Autodesk Inventor part; units mm, degrees
ref_plane "YZ Plane" through (0, 0, 0) normal (1, 0, 0) x (0, 1, 0)
ref_plane "XZ Plane" through (0, 0, 0) normal (0, 1, 0) x (-1, 0, 0)
ref_plane "XY Plane" through (0, 0, 0) normal (0, 0, 1) x (1, 0, 0)
sketch "Sketch2" plane through (0, 0, 0) normal (0, 0, 1) x (1, 0, 0)
  line L0 (-43.942, 43.18) -> (-43.942, 15.24)
  line L1 (-43.942, 15.24) -> (-36.322, 15.24)
  line L2 (-36.322, 15.24) -> (-25.4, 0)
  line L3 (-25.4, 0) -> (0, 0)
  line L4 (0, 0) -> (0, 43.18)
  line L5 (0.889, 43.18) -> (0.889, -1.778)
  line L6 (0.889, -1.778) -> (-45.72, -1.778)
  line L7 (-45.72, -1.778) -> (-45.72, 43.18)
  line L8 (-45.72, 43.18) -> (-43.942, 43.18)
  line L9 (0, 43.18) -> (0.889, 43.18)
  dimension "d1" = 7.62
  dimension "d2" = 27.94
  dimension "d3" = 10.922
  dimension "d4" = 43.18
  dimension "d5" = 1.778
  dimension "d6" = 0.889
  dimension "d7" = 1.778
  dimension "d10" = 44.958
  dimension "d11" = 46.609
extrude "Extrusion1" add sketch "Sketch2" along normal mid plane 20.828
sketch "Sketch5" plane through (0.889, -1.778, 10.414) normal (1, 0, 0) x (0, 0, -1)
  line L0 (0, 44.958) -> (20.828, 44.958)
  line L1 (3.175, 44.958) -> (17.653, 44.958)
  line L2 (17.653, 44.958) -> (17.653, 1.778)
  line L3 (17.653, 1.778) -> (3.175, 1.778)
  line L4 (3.175, 1.778) -> (3.175, 44.958)
  line L5 (0, 1.778) -> (20.828, 1.778)
  line L6 (0, 44.958) -> (20.828, 1.778) construction
  line L7 (3.175, 1.778) -> (17.653, 44.958) construction
  point P0 (10.414, 1.778)
  point P1 (10.414, 23.368)
  dimension "d14" = 14.478
extrude "Extrusion2" cut sketch "Sketch5" against normal up to next
sketch "Sketch6" plane through (0, 0, 10.414) normal (0, 0, 1) x (1, 0, 0)
  line L0 (-45.72, 43.18) -> (0.889, 43.18)
  line L1 (0.889, 43.18) -> (0.889, -1.778)
  line L2 (0.889, -1.778) -> (-45.72, -1.778)
  line L3 (-45.72, -1.778) -> (-45.72, 43.18)
extrude "Extrusion3" add sketch "Sketch6" along normal blind 0.889
mirror "Mirror1" about plane through (0, 0, 0) normal (0, 0, 1) of "Extrusion3"
properties part number "SteerServoInsert"
Geometry: final body of the model. Coordinates: model frame, mm. A direction names the side the tool comes from. Round coordinates to 2 decimals unless told otherwise and drop trailing zeros. Write each loop counter-clockwise with the first axis right and the second up, starting at its lowest first coordinate (ties: lowest second). Pieces come first, ordered by that corner, then holes. Notation, with made-up numbers: (11, 6) -> (27, 6) arc R25 cw to (27, 39) -> close; hole circle Ø9 at (-33.5, 12). An arc over 180 degrees is marked (long way). Use CSV: the item, a comma, the result in double quotes. Start each with the question number.
Q1. Section A-A (z = 9). Return loops of the section in (x, y).
Q2. Reachability of faces 4 (the face through (-22, 22, -10.414)), 5 (the face through (-22, 21, -11.303)) from +Z, -Z, +X, -X, +Y, -Y: full face, straight path, thin tool, end or side. Return the list, or none.
Q3. First-contact query: pin 1 Ø6 at (y, z) = (29, 4) entering from +X; pin 2 Ø4 at (x, z) = (-40.5, -0.5) entering from +Y. Flat tips, straight axial feed; report the tip coordinate or a pass-through.
Q4. Section C-C (x = -19). Return loops of the section in (y, z), plus the area to 3 significant figures.
Q5. Line query: L1, parallel to Z at x = -21, y = 38; L2, parallel to X at y = 24.5, z = 9.5; L3, parallel to X at y = 23.5, z = -7. Output: solid intervals per line, ascending.
Q6. Section D-D (z = 2.25). Return loops of the section in (x, y), plus the area to 3 significant figures.
Q7. Section B-B (y = 40). Return loops of the section in (x, z).
Q8. Pull-direction query (X, two-part tool) for faces 1 (the face through (-43.942, 29, 0)), 2 (the face through (0.889, 20, 8)), 3 (the face through (-23, -1.778, 0)); classes: pulls with the +X half, pulls with the -X half, needs draft (parallel to the pull), parting line crosses it, or undercut.
Result sheet:
1,outline,"(-45.72, -1.78) -> (0.89, -1.78) -> (0.89, 43.18) -> (0, 43.18) -> (0, 0) -> (-25.4, 0) -> (-36.32, 15.24) -> (-43.94, 15.24) -> (-43.94, 43.18) -> (-45.72, 43.18) -> close"
2,face 4,"+Y"
2,face 5,"-Z, +X, -X, +Y, -Y"
3,pin 1,"x = -43.94"
3,pin 2,"y = 15.24"
4,outline,"(-1.78, -11.3) -> (43.18, -11.3) -> (43.18, -10.41) -> (0, -10.41) -> (0, 10.41) -> (43.18, 10.41) -> (43.18, 11.3) -> (-1.78, 11.3) -> close"
4,area,"117 mm²"
5,L1,"-11.3 to -10.41, 10.41 to 11.3"
5,L2,"-45.72 to -43.94, 0 to 0.89"
5,L3,"-45.72 to -43.94"
6,outline,"(-45.72, -1.78) -> (0.89, -1.78) -> (0.89, 0) -> (-25.4, 0) -> (-36.32, 15.24) -> (-43.94, 15.24) -> (-43.94, 43.18) -> (-45.72, 43.18) -> close"
6,area,"359 mm²"
7,outline,"(-45.72, -11.3) -> (0.89, -11.3) -> (0.89, -7.24) -> (0, -7.24) -> (0, -10.41) -> (-43.94, -10.41) -> (-43.94, 10.41) -> (0, 10.41) -> (0, 7.24) -> (0.89, 7.24) -> (0.89, 11.3) -> (-45.72, 11.3) -> close"
8,face 1,"undercut"
8,face 2,"pulls with the +X half"
8,face 3,"needs draft"
